```python
from build123d import *

# Parameters (mm, degrees)
SKETCH1_W           = 43
SKETCH1_H           = 12
SKETCH1_R           = 1.5
BOSS_EXTRUDE1_DEPTH = 2
SKETCH2_W           = 43
SKETCH2_H           = 3
BOSS_EXTRUDE2_DEPTH = 13
SKETCH3_R           = 3.1
CUT_EXTRUDE1_DEPTH  = 13


with BuildPart() as part:
    # Sketch1 → Boss-Extrude1 (new body)
    with BuildSketch(Plane(origin=(0, 0, 0), x_dir=(1, 0, 0), z_dir=(0, 1, 0))):
        with Locations((-16.5, -1)):
            Rectangle(SKETCH1_W, SKETCH1_H)
        with Locations((-33, 0)):
            Circle(SKETCH1_R, mode=Mode.SUBTRACT)
        Circle(SKETCH1_R, mode=Mode.SUBTRACT)
    extrude(amount=BOSS_EXTRUDE1_DEPTH)

    # Sketch2 → Boss-Extrude2 (add)
    with BuildSketch(Plane(origin=(0, 2, 0), x_dir=(1, 0, 0), z_dir=(0, 1, 0))):
        with Locations((-16.5, -5.5)):
            Rectangle(SKETCH2_W, SKETCH2_H)
    extrude(amount=BOSS_EXTRUDE2_DEPTH)

    # Sketch3 → Cut-Extrude1 (cut)
    with BuildSketch(Plane.XY.offset(7)):
        with Locations((-27.25, 8.5)):
            Circle(SKETCH3_R)
        with Locations((-5.75, 8.5)):
            Circle(SKETCH3_R)
    extrude(amount=-CUT_EXTRUDE1_DEPTH, mode=Mode.SUBTRACT)


solid = part.part
```
Geometry: final body of the model. Coordinates: model frame, mm. A direction names the side the tool comes from. Coordinates: 2 decimals unless noted, no trailing zeros. Order: outer loops, then holes, each group sorted by start corner. A loop starts at its lowest first (then second) coordinate and runs counter-clockwise, first axis right, second up. Notation, with made-up numbers: M 40.25,-5.75 L 97.25,-5.75 A35 ccw 97.25,29.25 Z; hole C -28,54 d11. An arc over 180 degrees is marked long. Answer in a Markdown table with one row per item. Add a question column.
Q1. Line query: L1, parallel to X at y = 1.2, z = 0; L2, parallel to Y at x = -27.25, z = 5.65; L3, parallel to Z at x = 0, y = 0.65. Output: solid intervals per line, ascending.
Q2. Reachability of faces 4 (the flat face through (-17, 8, 4)), 5 (the cylindrical face through (-30.347, 8.636, 5.521)) from +Z, -Z, +X, -X, +Y, -Y: full face, straight path, thin tool, end or side. Return the list, or none.
Q3. Mould query, pull axis Z, two halves, no side actions, for faces 1 (the flat face through (-17, 1, -5)), 2 (the cylindrical face through (-34.2, 1, 0.9)), 3 (the flat face through (-17, 15, 5)). Classes: released by +Z, released by -Z, zero draft, split by the parting line, or undercut.
Q4. Section query A-A on x = -27.25. Return the cut outline in (y, z), and give its area (3 significant figures).
Q5. Section query D-D on z = 5. Return the cut outline in (x, y).
Q6. Section query C-C on y = 8.5. Return the cut outline in (x, z), and give its area (3 significant figures).
Q7. Contact query for flat-ended pins moving along their axis: P1, Ø2.5, axis at x = 0, z = 0, coming from the +Y side; P2, Ø4.5, axis at x = -11.5, z = -0.5, coming from the +Y side; P3, Ø6, axis at y = 4, z = 2.5, coming from the -X side; P4, Ø6.5, axis at x = -18.5, y = 6, coming from the -Z side. Output: stop coordinate, or through.
Q8. Section query B-B on z = 0. Return the cut outline in (x, y), and give its area (3 significant figures).
Completed:
| question | item | result |
|---|---|---|
| 1 | L1 | x = -38 to -34.5, -31.5 to -1.5, 1.5 to 5 |
| 1 | L2 | y = 0 to 5.4, 11.6 to 15 |
| 1 | L3 | z = -5 to -1.5, 1.5 to 7 |
| 2 | face 4 | -Z, +X, -X, +Y |
| 2 | face 5 | +Z, -Z |
| 3 | face 1 | released by -Z |
| 3 | face 2 | undercut |
| 3 | face 3 | zero draft |
| 4 | outline | M 0,-5 L 2,-5 L 2,4 L 5.4,4 L 5.4,7 L 0,7 Z; M 11.6,4 L 15,4 L 15,7 L 11.6,7 Z |
| 4 | area | 44.4 mm2 |
| 5 | outline | M -38,0 L 5,0 L 5,15 L -38,15 Z; hole C -27.25,8.5 d6.2; hole C -5.75,8.5 d6.2 |
| 6 | outline | M -38,4 L -30.35,4 L -30.35,7 L -38,7 Z; M -24.15,4 L -8.85,4 L -8.85,7 L -24.15,7 Z; M -2.65,4 L 5,4 L 5,7 L -2.65,7 Z |
| 6 | area | 91.8 mm2 |
| 7 | P1 | passes through |
| 7 | P2 | stops at y = 2 |
| 7 | P3 | stops at x = -38 |
| 7 | P4 | stops at z = 4 |
| 8 | outline | M -38,0 L -34.5,0 L -34.5,2 L -38,2 Z; M -31.5,0 L -1.5,0 L -1.5,2 L -31.5,2 Z; M 1.5,0 L 5,0 L 5,2 L 1.5,2 Z |
| 8 | area | 74.0 mm2 |
